```python
from build123d import *

# Parameters (mm, degrees)
RIBCUT1_DEPTH    = 0.28575
RIBCUT2_DEPTH    = 0.4572
RIBCUTSPAT_COUNT = 12
RIBCUTSPAT_ANGLE = 330


with BuildPart() as part:
    # BodySke → BaseBody (revolve)
    with BuildSketch(Plane.XY):
        with BuildLine():
            Line((0, 0), (0, 2.77876))
            Line((0, 2.77876), (0.00508, 2.77876))
            Line((0.00508, 2.77876), (0.00508, 2.78384))
            ThreePointArc((0.00508, 2.78384), (0.23114, 3.0099), (0.4572, 2.78384))
            Line((0.4572, 2.78384), (0.4572, 2.7178))
            Line((0.4572, 2.7178), (0.9144, 2.4003))
            Line((0.9144, 2.4003), (0.9144, 2.0828))
            Line((0.9144, 2.0828), (18.57756, 2.0828))
            Line((18.57756, 2.0828), (19.05, 1.61036))
            Line((19.05, 1.61036), (19.05, 0))
            Line((19.05, 0), (0, 0))
        make_face()
    revolve(axis=Axis((0, 0, 0), (1, 0, 0)))

    # RibCut1Ske → RibCut1 (cut)
    with BuildSketch(Plane(origin=(0.9144, 0, 0), x_dir=(0, 0, -1), z_dir=(1, 0, 0))):
        with BuildLine():
            Line((0.271859953, 2.064981357), (0.271859953, 2.997597401))
            ThreePointArc((0.271859953, 2.997597401), (0.779019444, 2.907340145), (1.263361075, 2.731925476))
            Line((1.263361075, 2.731925476), (0.797053053, 1.92425629))
            ThreePointArc((0.797053053, 1.92425629), (0.539068307, 2.011830311), (0.271859953, 2.064981357))
        make_face()
    ribcut1 = extrude(amount=-RIBCUT1_DEPTH, mode=Mode.SUBTRACT)

    # RibCut2Ske → RibCut2 (cut)
    with BuildSketch(Plane(origin=(0.9144, 0, 0), x_dir=(0, 0, -1), z_dir=(1, 0, 0))):
        with BuildLine():
            Line((0.271859953, 2.384854766), (0.271859953, 2.997597401))
            ThreePointArc((0.271859953, 2.997597401), (0.779019444, 2.907340145), (1.263361075, 2.731925476))
            Line((1.263361075, 2.731925476), (0.956989757, 2.201274788))
            ThreePointArc((0.956989757, 2.201274788), (0.621243354, 2.318511761), (0.271859953, 2.384854766))
        make_face()
    ribcut2 = extrude(amount=-RIBCUT2_DEPTH, mode=Mode.SUBTRACT)

    # RibCutsPat: RibCut1, RibCut2 ×12 about axis
    ribcutspat_axis = Axis((0, 0, 0), (1, 0, 0))
    for i in range(1, RIBCUTSPAT_COUNT):
        add(ribcut1.rotate(ribcutspat_axis, i * RIBCUTSPAT_ANGLE / (RIBCUTSPAT_COUNT - 1)), mode=Mode.SUBTRACT)
        add(ribcut2.rotate(ribcutspat_axis, i * RIBCUTSPAT_ANGLE / (RIBCUTSPAT_COUNT - 1)), mode=Mode.SUBTRACT)


solid = part.part
```
Model file for the job. Use its own axes, mm. Coordinates: 2 decimals unless noted, no trailing zeros. Order: outer loops, then holes, each group sorted by start corner. A loop starts at its lowest first (then second) coordinate and runs counter-clockwise, first axis right, second up. Notation, with made-up numbers: (-29.75, 64) -> (-19.75, 64) arc R19 cw to (-19.75, 87) -> close; hole circle Ø4 at (-0.5, 72). An arc over 180 degrees is marked (long way). Return JSON: item names as keys, results as strings.
Item 1: Pin check, flat tips, straight feed: P1, Ø0.5, axis at y = 0.5, z = 2, coming from the +X side; P2, Ø0.7, axis at y = -1.5, z = 1.5, coming from the +X side; P3, Ø3, axis at x = 14.5, y = -0.5, coming from the +Z side. Stop position of each tip, or through.
Model answer:
{"P1": "stops at x = 18.85", "P2": "stops at x = 18.89", "P3": "stops at z = 2.08"}
Item 2: Wall check: line 1 along X through (y, z) = (1.5, -1.5); line 2 along Y through (x, z) = (1.75, -0.25); line 3 along X through (y, z) = (-1, -2.5). Give the ranges that are in metal, low to high. Write a range as from..to.
Model answer:
{"line 1": "x = 0..0.63", "line 2": "y = -2.07..2.07", "line 3": "x = 0..0.46"}
Item 3: Slice it at C-C (x = 5.25). Write the cut outline in (y, z).
Model answer:
{"outline": "circle Ø4.17 at (0, 0)"}
